The model under review builds one solid part; all positions refer to its coordinate system, in mm. A direction names the side the tool comes from. Coordinates: 2 decimals unless noted, no trailing zeros. Order: outer loops, then holes, each group sorted by start corner. A loop starts at its lowest first (then second) coordinate and runs counter-clockwise, first axis right, second up. Notation, with made-up numbers: (52, 0) - (56, 0) arc R23 cw to (56, 21) - close; hole circle Ø6 at (45, 39.25). An arc over 180 degrees is marked (long way). Answer in a Markdown table with one row per item.
```python
from build123d import *

# Parameters (mm, degrees)
PRISM_DEPTH             = 4
PRISM_PITCH_ANGLE       = 90
CYLINDER_R              = 1.7
CYLINDER_DEPTH          = 20
CYLINDER_PITCH_ANGLE    = 90
CYLINDER001_R           = 4.9
CYLINDER001_DEPTH       = 3
CYLINDER001_PITCH_ANGLE = 90
PAD_DEPTH               = 10
PAD001_DEPTH            = 2
POCKET_DEPTH            = 5


with BuildPart() as prisma:
    # Prism → Prism (new body)
    with BuildSketch(Plane.XY):
        Polygon((3.1, 0), (1.55, 2.684679), (-1.55, 2.684679), (-3.1, 0), (-1.55, -2.684679), (1.55, -2.684679), align=None)
    extrude(amount=PRISM_DEPTH)


with BuildPart() as prisma_1:
    # Prism pitch: moved
    add(prisma.part.rotate(Axis((0, 0, 0), (0, 1, 0)), PRISM_PITCH_ANGLE))


with BuildPart() as prisma_2:
    # Prism placement: moved
    add(prisma_1.part.moved(Location((13, 32, 5))))


with BuildPart() as cilindro:
    # Cylinder → Cylinder (new body)
    with BuildSketch(Plane.XY):
        Circle(CYLINDER_R)
    extrude(amount=CYLINDER_DEPTH)


with BuildPart() as cilindro_1:
    # Cylinder pitch: moved
    add(cilindro.part.rotate(Axis((0, 0, 0), (0, 1, 0)), CYLINDER_PITCH_ANGLE))


with BuildPart() as cilindro_2:
    # Cylinder placement: moved
    add(cilindro_1.part.moved(Location((-4, 32, 5))))


with BuildPart() as cilindro001:
    # Cylinder001 → Cylinder001 (new body)
    with BuildSketch(Plane.XY):
        Circle(CYLINDER001_R)
    extrude(amount=CYLINDER001_DEPTH)


with BuildPart() as cilindro001_1:
    # Cylinder001 pitch: moved
    add(cilindro001.part.rotate(Axis((0, 0, 0), (0, 1, 0)), CYLINDER001_PITCH_ANGLE))


with BuildPart() as cilindro001_2:
    # Cylinder001 placement: moved
    add(cilindro001_1.part.moved(Location((12.5, 32, 5))))


with BuildPart() as pocket:
    # Sketch → Pad (new body)
    with BuildSketch(Plane.XY):
        with BuildLine():
            Line((0, 40), (0, 0))
            Line((0, 0), (2.5, 0))
            Line((2.5, 0), (2.5, 40))
            ThreePointArc((11.5, 40), (7, 44.5), (2.5, 40))
            Line((11.5, 40), (11.5, 25))
            Line((11.5, 25), (14, 25))
            Line((14, 25), (14, 40))
            ThreePointArc((14, 40), (7, 47), (0, 40))
        make_face()
    extrude(amount=PAD_DEPTH)

    # Fusion: union Cilindro001
    add(cilindro001_2.part)

    # Cut: cut Cilindro
    add(cilindro_2.part, mode=Mode.SUBTRACT)

    # Cut001: cut Prisma
    add(prisma_2.part, mode=Mode.SUBTRACT)

    # Sketch001 → Pad001 (new body, symmetric)
    with BuildSketch(Plane(origin=(0, 0, 0), x_dir=(0, -1, 0), z_dir=(-1, 0, 0))):
        with BuildLine():
            ThreePointArc((-22.000056, 10), (-27.000056, 4.999986), (-22.000028, 0))
            Line((-22.000028, 0), (-5.000028, 0))
            ThreePointArc((-5.000028, 0), (0, 4.999986), (-5, 10))
            Line((-22.000056, 10), (-5, 10))
        make_face()
    extrude(amount=PAD001_DEPTH, both=True)

    # Sketch002 → Pocket (cut)
    with BuildSketch(Plane(origin=(-2, 0, 0), x_dir=(0, -1, 0), z_dir=(-1, 0, 0))):
        with BuildLine():
            ThreePointArc((-21.99998, 7.5), (-24.499981, 5.00001), (-22, 2.5))
            Line((-22, 2.5), (-5, 2.5))
            ThreePointArc((-5, 2.5), (-2.500017, 5.000009), (-5.000017, 7.5))
            Line((-21.99998, 7.5), (-5.000017, 7.5))
        make_face()
    extrude(amount=-POCKET_DEPTH, mode=Mode.SUBTRACT)


solid = pocket.part
```
Item 1: Tool access review of faces 4 (the face through (0.22, 2.5, 4.95)), 5 (the face through (2.5, 20, 2)), 6 (the face through (0, 1, 9)): name each direction out of +Z, -Z, +X, -X, +Y, -Y from which nothing blocks a thin tool from reaching the whole face with its end or side.
Check values:
| item | result |
|---|---|
| face 4 | +X, -X |
| face 5 | +Z, -Z, -Y |
| face 6 | +Z, -X, -Y |
Item 2: We need section D-D, the plane z = 8.75. Write out the cut boundary in (x, y), then the cut area to 3 significant figures.
Check values:
| item | result |
|---|---|
| outline | (-2, 1.69) - (0, 1.69) - (0, 0) - (2.5, 0) - (2.5, 40) arc R4.5 cw to (11.5, 40) - (11.5, 25) - (14, 25) - (14, 28.85) - (15.5, 28.85) - (15.5, 35.15) - (14, 35.15) - (14, 40) arc R7 ccw to (0, 40) - (0, 25.31) - (-2, 25.31) - close |
| area | 239 mm^2 |
Item 3: We need section A-A, the plane y = 12. Write out the cut boundary in (x, z).
Check values:
| item | result |
|---|---|
| outline | (-2, 0) - (2.5, 0) - (2.5, 2.5) - (-2, 2.5) - close; (-2, 7.5) - (2.5, 7.5) - (2.5, 10) - (-2, 10) - close |
Item 4: To check wall thickness, follow line 1 (Z direction, x = 12, y = 32); line 2 (X direction, y = 29.5, z = 5); line 3 (X direction, y = 26, z = 8.75). State the ranges of each line that lie inside material, in increasing order. Write a range as from..to.
Check values:
| item | result |
|---|---|
| line 1 | 0..3.3, 6.7..10 |
| line 2 | 0..2.5, 11.5..13 |
| line 3 | 0..2.5, 11.5..14 |
Item 5: Mouldability with a two-part tool opening along Y and no side actions: class faces 1 (the face through (2, 25, 10)), 2 (the face through (-1, 0, 5)), 3 (the face through (0, 14, 7.5)) as +Y half, -Y half, draft (parallel to the pull), parting line (faces both ways), or undercut.
Check values:
| item | result |
|---|---|
| face 1 | draft |
| face 2 | -Y half |
| face 3 | undercut |
Item 6: We need section C-C, the plane x = 12.5. Write out the cut boundary in (y, z), then the cut area to 3 significant figures.
Check values:
| item | result |
|---|---|
| outline | (25, 0) - (44.33, 0) - (44.33, 10) - (25, 10) - close; hole circle Ø3.4 at (32, 5) |
| area | 184 mm^2 |
Item 7: Clearance check with flat-ended pins moving along their axes: pin 1 Ø1.5 at (y, z) = (40.5, 8) entering from +X; pin 2 Ø3 at (y, z) = (32, 6.5) entering from -X; pin 3 Ø2 at (x, z) = (14, 5.5) entering from -Y. State where each tip first meets the part, or that it passes through.
Check values:
| item | result |
|---|---|
| pin 1 | x = 14 |
| pin 2 | x = 0 |
| pin 3 | y = 25 |
Item 8: We need section B-B, the plane z = 4. State how many separate pieces and enclosed holes the cut face has, then the cut area to 3 significant figures.
Check values:
| item | result |
|---|---|
| separate pieces | 4 |
| enclosed holes | 0 |
| area | 129 mm^2 |
